Autodesk Inventor part; units mm, degrees
ref_plane "YZ Plane" through (0, 0, 0) normal (1, 0, 0) x (0, 1, 0)
ref_plane "XZ Plane" through (0, 0, 0) normal (0, 1, 0) x (-1, 0, 0)
ref_plane "XY Plane" through (0, 0, 0) normal (0, 0, 1) x (1, 0, 0)
sketch "Sketch1" plane through (0, 0, 0) normal (0, 1, 0) x (-1, 0, 0)
  circle A0 centre (0, 0) radius 2
  dimension "d0" = 4
extrude "Extrusion1" add sketch "Sketch1" along normal blind 12
sketch "Sketch2" plane through (0, 12, 0) normal (0, 1, 0) x (1, 0, 0)
  circle A0 centre (0, 0) radius 2
  circle A1 centre (0, 0) radius 3.5
  dimension "d3" = 7
extrude "Extrusion2" add sketch "Sketch2" along normal blind 4 contours A0 | A1
sketch "Sketch3" plane through (0, 16, 0) normal (0, 1, 0) x (1, 0, 0)
  circle A0 centre (0, 0) radius 3.5
  line L0 (0, 1.8475) -> (1.6, 0.9238)
  line L1 (1.6, 0.9238) -> (1.6, -0.9238)
  line L2 (1.6, -0.9238) -> (0, -1.8475)
  line L3 (0, -1.8475) -> (-1.6, -0.9238)
  line L4 (-1.6, -0.9238) -> (-1.6, 0.9238)
  line L5 (-1.6, 0.9238) -> (0, 1.8475)
  dimension "d6" = 1.6
extrude "Extrusion3" cut sketch "Sketch3" against normal blind 3 contours L0 L1 L2 L3 L4 L5
thread "Thread1"
chamfer "Chamfer1" distance 0.25 angle 45 1 edges at (2, 0, 0)
properties part number "SHCS4x12"
Model file for the job. Use its own axes, mm. A direction names the side the tool comes from. Give positions to 0.01 mm unless a question says otherwise; leave off trailing zeros. Loops run counter-clockwise (first coordinate to the right, second up) from the corner with the lowest first, then second, coordinate; pieces in that order, holes last. Notation, with made-up numbers: (86, 15.25) - (108, 15.25) arc R15 ccw to (108, 38.25) - close; hole circle Ø4 at (26.5, 20). An arc over 180 degrees is marked (long way). Use one line per item in the form item = value.
(1) Cut at D-D (x = 3). Give the cut face in (y, z).
Determined:
outline = (12, -1.8) - (16, -1.8) - (16, 1.8) - (12, 1.8) - close
(2) Cut at A-A (y = 14.5). Give the cut face in (x, z).
Determined:
outline = circle Ø7 at (0, 0); hole (-1.6, -0.92) - (0, -1.85) - (1.6, -0.92) - (1.6, 0.92) - (0, 1.85) - (-1.6, 0.92) - close
(3) Pull direction X, two halves, no side cores. Call faces 4 (the face through (-0.79, 14.52, 1.39)), 5 (the face through (-2, 16, 0)), 6 (the face through (3.233, 13.972, -1.341)): pulls with the +X half, pulls with the -X half, needs draft (parallel to the pull), parting line crosses it, or undercut.
Determined:
face_4 = undercut
face_5 = needs draft
face_6 = parting line crosses it
(4) 3-axis set-ups, long thin cutter, end or side, ignore diameter. For faces 1 (the face through (0, 0, 0)), 2 (the face through (0, 6, 2)), 3 (the face through (-1.6, 15, 0)): which of +Z, -Z, +X, -X, +Y, -Y reach the whole face in a straight line?
Determined:
face_1 = +Z, -Z, +X, -X, -Y
face_2 = -Y
face_3 = +Y
(5) Drill centre lines: L1, parallel to Y at x = 0.5, z = -3; L2, parallel to Z at x = 1.25, y = 11; L3, parallel to Z at x = -0.25, y = 1. Where is each one in solid material? Low to high.
Determined:
L1 = 12 to 16
L2 = -1.56 to 1.56
L3 = -1.98 to 1.98
(6) Cut at B-B (z = 0). Give the cut face in (x, y).
Determined:
outline = (-3.5, 12) - (-2, 12) - (-2, 0.25) - (-1.75, 0) - (1.75, 0) - (2, 0.25) - (2, 12) - (3.5, 12) - (3.5, 16) - (1.6, 16) - (1.6, 13) - (-1.6, 13) - (-1.6, 16) - (-3.5, 16) - close
(7) Cut at C-C (y = 4.5). Give the cut face in (x, z), then the cut area to 3 significant figures.
Determined:
outline = circle Ø4 at (0, 0)
area = 12.6 mm^2
(8) Drop flat-ended pins along their axis: P1, Ø1.5, axis at x = 2.5, y = 6, coming from the -Z side; P2, Ø2, axis at y = 12, z = -2, coming from the -X side; P3, Ø1.5, axis at y = 5, z = 1.5, coming from the +X side. Give the stop position or say it passes through.
Determined:
P1 = -0.97
P2 = -3.35
P3 = 1.85
